Geometry check sheet. Reference: the model listing, model coordinates, mm. Round coordinates to 2 decimals unless told otherwise and drop trailing zeros. Write each loop counter-clockwise with the first axis right and the second up, starting at its lowest first coordinate (ties: lowest second). Pieces come first, ordered by that corner, then holes. Notation, with made-up numbers: (33, 85.25) -> (61, 85.25) arc R17 cw to (61, 98.25) -> close; hole circle Ø8 at (17, 34). An arc over 180 degrees is marked (long way). Use a Markdown table: item, result.
Autodesk Inventor part; units mm, degrees
ref_plane "YZ Plane" through (0, 0, 0) normal (1, 0, 0) x (0, 1, 0)
ref_plane "XZ Plane" through (0, 0, 0) normal (0, 1, 0) x (-1, 0, 0)
ref_plane "XY Plane" through (0, 0, 0) normal (0, 0, 1) x (1, 0, 0)
sketch "Sketch1" plane through (0, 0, 0) normal (0, 0, 1) x (1, 0, 0)
  line L0 (0, 0) -> (355.6, 0) construction
  line L1 (355.6, 0) -> (355.6, 50.8) construction
  line L2 (355.6, 50.8) -> (0, 50.8) construction
  line L3 (0, 50.8) -> (0, 0) construction
  line L4 (57.1297, 50.8) -> (304.8, 404.5099) construction
  line L5 (304.8, 404.5099) -> (325.6065, 389.941) construction
  line L6 (325.6065, 389.941) -> (77.9362, 36.2312) construction
  line L7 (77.9362, 36.2312) -> (57.1297, 50.8) construction
  line L8 (355.6, 50.8) -> (304.8, 50.8) construction
  line L9 (304.8, 50.8) -> (304.8, 438.15) construction
  line L10 (304.8, 438.15) -> (355.6, 438.15) construction
  line L11 (355.6, 438.15) -> (355.6, 50.8) construction
  line L12 (57.15, 75.8737) -> (95.25, 75.8737)
  line L13 (95.25, 75.8737) -> (95.25, 0)
  line L14 (95.25, 0) -> (57.15, 0)
  line L15 (57.15, 0) -> (57.15, 75.8737)
  line L16 (320.675, 41.275) -> (288.925, 41.275) construction
  line L17 (288.925, 41.275) -> (288.925, 9.525) construction
  line L18 (288.925, 9.525) -> (320.675, 9.525) construction
  line L19 (320.675, 9.525) -> (320.675, 41.275) construction
  line L20 (234.95, 41.275) -> (203.2, 41.275) construction
  line L21 (203.2, 41.275) -> (203.2, 9.525) construction
  line L22 (203.2, 9.525) -> (234.95, 9.525) construction
  line L23 (234.95, 9.525) -> (234.95, 41.275) construction
  line L24 (67.5329, 43.5156) -> (111.2395, 105.935) construction
  circle A0 centre (63.5, 42.8625) radius 2.5527 construction
  line L25 (74.6865, 75.8737) -> (57.1297, 50.8)
  point P0 (88.1374, 50.8)
  point P1 (342.9, 42.8625)
  point P2 (330.2, 25.4)
  point P3 (342.9, 7.9375)
  point P4 (355.6, 25.4)
  point P5 (317.5, 42.8625)
  point P6 (304.8, 25.4)
  point P7 (317.5, 7.9375)
  point P8 (292.1, 42.8625)
  point P9 (279.4, 25.4)
  point P10 (292.1, 7.9375)
  point P11 (266.7, 42.8625)
  point P12 (254, 25.4)
  point P13 (266.7, 7.9375)
  point P14 (241.3, 42.8625)
  point P15 (228.6, 25.4)
  point P16 (241.3, 7.9375)
  point P17 (215.9, 42.8625)
  point P18 (203.2, 25.4)
  point P19 (215.9, 7.9375)
  point P20 (190.5, 42.8625)
  point P21 (177.8, 25.4)
  point P22 (190.5, 7.9375)
  point P23 (165.1, 42.8625)
  point P24 (152.4, 25.4)
  point P25 (165.1, 7.9375)
  point P26 (139.7, 42.8625)
  point P27 (127, 25.4)
  point P28 (139.7, 7.9375)
  point P29 (114.3, 42.8625)
  point P30 (101.6, 25.4)
  point P31 (114.3, 7.9375)
  point P32 (88.9, 42.8625)
  point P33 (76.2, 25.4)
  point P34 (88.9, 7.9375)
  point P35 (50.8, 25.4)
  point P36 (63.5, 7.9375)
  point P37 (38.1, 42.8625)
  point P38 (25.4, 25.4)
  point P39 (38.1, 7.9375)
  point P40 (12.7, 42.8625)
  point P41 (0, 25.4)
  point P42 (12.7, 7.9375)
  point P43 (-12.7, 42.8625)
  point P44 (-25.4, 25.4)
  point P45 (-12.7, 7.9375)
  point P46 (320.675, 25.4)
  point P47 (234.95, 25.4)
  point P48 (288.925, 25.4)
  point P49 (78.4596, 59.1204)
  point P50 (85.744, 69.5237)
  point P51 (93.0284, 79.9269)
  point P52 (100.3128, 90.3301)
  point P53 (57.15, 50.829)
  dimension "d0" = 50.8
  dimension "d1" = 355.6
  dimension "d2" = 55
  dimension "d3" = 25.4
  dimension "d4" = 50.8
  dimension "d5" = 387.35
  dimension "d6" = 431.8
  dimension "d10" = 12.7
  dimension "d11" = 7.9375
  dimension "d12" = 25.4
  dimension "d13" = 7.9375
  dimension "d16" = 25.4
  dimension "d21" = 34.925
  dimension "d22" = 31.75
  dimension "d23" = 31.75
  dimension "d24" = 31.75
  dimension "d25" = 120.65
  dimension "d26" = 31.75
  dimension "d27" = 76.2
  dimension "d28" = 19.05
  dimension "d31" = 12.7
  dimension "d37" = 6.35
  dimension "d38" = 6.35
  dimension "d39" = 6.35
  dimension "d40" = 5.1054
extrude "Extrusion1" add sketch "Sketch1" against normal blind 6.35 contours L12 L13 L14 L15 L25
hole "Hole1" at (342.9, 42.8625, 0) at (330.2, 25.4, 0) at (342.9, 7.9375, 0) at (317.5, 42.8625, 0) at (304.8, 25.4, 0) at (317.5, 7.9375, 0) at (292.1, 42.8625, 0) at (279.4, 25.4, 0) at (292.1, 7.9375, 0) at (266.7, 42.8625, 0) at (254, 25.4, 0) at (266.7, 7.9375, 0) at (241.3, 42.8625, 0) at (228.6, 25.4, 0) at (241.3, 7.9375, 0) at (215.9, 42.8625, 0) at (203.2, 25.4, 0) at (215.9, 7.9375, 0) at (190.5, 42.8625, 0) at (177.8, 25.4, 0) at (190.5, 7.9375, 0) at (165.1, 42.8625, 0) at (152.4, 25.4, 0) at (165.1, 7.9375, 0) at (139.7, 42.8625, 0) at (127, 25.4, 0) at (139.7, 7.9375, 0) at (114.3, 42.8625, 0) at (101.6, 25.4, 0) at (114.3, 7.9375, 0) at (88.9, 42.8625, 0) at (76.2, 25.4, 0) at (88.9, 7.9375, 0) at (63.5, 42.8625, 0) at (50.8, 25.4, 0) at (63.5, 7.9375, 0) at (38.1, 42.8625, 0) at (25.4, 25.4, 0) at (38.1, 7.9375, 0) at (12.7, 42.8625, 0) at (0, 25.4, 0) at (12.7, 7.9375, 0) at (-12.7, 42.8625, 0) at (-25.4, 25.4, 0) at (-12.7, 7.9375, 0) at (78.4596, 59.1204, 0) at (85.744, 69.5237, 0) at (93.0284, 79.9269, 0) at (100.3128, 90.3301, 0) direction (0, 0, -1) diameter 3.9624 end through all
fillet "Fillet1" radius 3.175 5 edges at (57.15, 0, -3.175) (95.25, 0, -3.175) (57.15, 50.829, -3.175) (74.6865, 75.8737, -3.175) (95.25, 75.8737, -3.175)
equation "\"d23\" = d22"
equation "\"d24\" = d22"
equation "\"d26\" = d22"
properties part number "CL7-012" material "Aluminum 6061"
(1) Section check A-A on x = 88.9. Record the cut outline in (y, z), plus the area to 3 significant figures.
A:
| item | result |
|---|---|
| outline | (0, -6.35) -> (5.96, -6.35) -> (5.96, 0) -> (0, 0) -> close; (9.92, -6.35) -> (40.88, -6.35) -> (40.88, 0) -> (9.92, 0) -> close; (44.84, -6.35) -> (75.87, -6.35) -> (75.87, 0) -> (44.84, 0) -> close |
| area | 431 mm2 |
(2) Section check C-C on z = -5.5. State how many separate pieces and enclosed holes the cut face has, plus the area to 3 significant figures.
A:
| item | result |
|---|---|
| separate pieces | 1 |
| enclosed holes | 7 |
| area | 2,580 mm2 |
(3) Thickness scan on line 1 (X direction, y = 8.5, z = -2.25); line 2 (Y direction, x = 63.5, z = -1.75); line 3 (Y direction, x = 64, z = -1.75). Record the ranges inside material, lowest first.
A:
| item | result |
|---|---|
| line 1 | x = 57.15 to 61.6, 65.4 to 87, 90.8 to 95.25 |
| line 2 | y = 0 to 5.96, 9.92 to 40.88, 44.84 to 59.9 |
| line 3 | y = 0 to 6.02, 9.85 to 40.95, 44.78 to 60.61 |
(4) Release check for a two-part mould opening along X. For faces 1 (the face through (57.15, 26, -3)), 2 (the face through (80.394, 59.55, -3.219)), 3 (the face through (84, 75.874, -3)), 4 (the face through (95.25, 38, -3)) record: +X half, -X half, draft (parallel to the pull), parting line (faces both ways), or undercut.
A:
| item | result |
|---|---|
| face 1 | -X half |
| face 2 | undercut |
| face 3 | draft |
| face 4 | +X half |
(5) Section check B-B on y = 25.4. Record the cut outline in (x, z), plus the area to 3 significant figures.
A:
| item | result |
|---|---|
| outline | (57.15, -6.35) -> (74.22, -6.35) -> (74.22, 0) -> (57.15, 0) -> close; (78.18, -6.35) -> (95.25, -6.35) -> (95.25, 0) -> (78.18, 0) -> close |
| area | 217 mm2 |
(6) Section check D-D on x = 64.5. Record the cut outline in (y, z).
A:
| item | result |
|---|---|
| outline | (0, -6.35) -> (6.23, -6.35) -> (6.23, 0) -> (0, 0) -> close; (9.65, -6.35) -> (41.15, -6.35) -> (41.15, 0) -> (9.65, 0) -> close; (44.57, -6.35) -> (61.33, -6.35) -> (61.33, 0) -> (44.57, 0) -> close |
(7) Gauge pin test, flat ends, axial feed: pin 1 Ø5 at (x, y) = (77.5, 19.5) entering from +Z; pin 2 Ø3 at (x, y) = (63.5, 7.94) entering from -Z. Record the tip position at first contact, or that the pin passes through.
A:
| item | result |
|---|---|
| pin 1 | stops at z = 0 |
| pin 2 | passes through |
